from build123d import *

# Parameters (mm, degrees)
SKETCH1_R                      = 63.5
BOSS_EXTRUDE1_DEPTH            = 3.175
SKETCH2_R                      = 12.9
BOSS_EXTRUDE2_DEPTH            = 3.175
BOSS_EXTRUDE3_START            = 3.175
SKETCH3_R                      = 63.5
SKETCH3_R_2                    = 25.4
BOSS_EXTRUDE3_DEPTH            = 3.175
SKETCH5_R                      = 10.4
CUT_EXTRUDE1_DEPTH             = 2.35
SKETCH6_R                      = 5
CUT_EXTRUDE2_DEPTH             = 4
CBORE_FOR_M2_SHCS1_D           = 2.2
CBORE_FOR_M2_SHCS1_DEPTH       = 6
CBORE_FOR_M2_SHCS1_CBORE_D     = 4.4
CBORE_FOR_M2_SHCS1_CBORE_DEPTH = 2
CBORE_FOR_M2_SHCS1_TIP         = 0.660946681


with BuildPart() as part:
    # Sketch1 → Boss-Extrude1 (new body)
    with BuildSketch(Plane(origin=(0, 0, 0), x_dir=(1, 0, 0), z_dir=(0, 1, 0))):
        with Locations(Location((0, 0, 0), (0, 0, 270))):
            Circle(SKETCH1_R)
    extrude(amount=BOSS_EXTRUDE1_DEPTH)

    # Sketch2 → Boss-Extrude2 (add)
    with BuildSketch(Plane.XZ):
        with Locations(Location((0, 0, 0), (0, 0, 270))):
            Circle(SKETCH2_R)
    extrude(amount=BOSS_EXTRUDE2_DEPTH)

    # Sketch3 → Boss-Extrude3 (add)
    with BuildSketch(Plane.XZ.offset(BOSS_EXTRUDE3_START)):
        with Locations(Location((0, 0, 0), (0, 0, 270))):
            Circle(SKETCH3_R)
        with Locations(Location((0, 0, 0), (0, 0, 270))):
            Circle(SKETCH3_R_2, mode=Mode.SUBTRACT)
    extrude(amount=-BOSS_EXTRUDE3_DEPTH)

    # Sketch5 → Cut-Extrude1 (cut)
    with BuildSketch(Plane(origin=(0, 3.175, 0), x_dir=(1, 0, 0), z_dir=(0, 1, 0))):
        with Locations(Location((0, 0, 0), (0, 0, 270))):
            Circle(SKETCH5_R)
    extrude(amount=-CUT_EXTRUDE1_DEPTH, mode=Mode.SUBTRACT)

    # Sketch6 → Cut-Extrude2 (cut)
    with BuildSketch(Plane(origin=(0, 0.825, 0), x_dir=(1, 0, 0), z_dir=(0, 1, 0))):
        with Locations(Location((0, 0, 0), (0, 0, 270))):
            Circle(SKETCH6_R)
    extrude(amount=-CUT_EXTRUDE2_DEPTH, mode=Mode.SUBTRACT)

    # CBORE for M2 SHCS1
    with Locations(Plane(origin=(0, 0.825, 0), x_dir=(1, 0, 0), z_dir=(0, 1, 0))):
        with Locations((-5.65685425, 5.65685425), (0, 8), (5.65685425, 5.65685425), (8, 0), (5.65685425, -5.65685425), (0, -8), (-5.65685425, -5.65685425), (-8, 0)):
            CounterBoreHole(CBORE_FOR_M2_SHCS1_D / 2, CBORE_FOR_M2_SHCS1_CBORE_D / 2, CBORE_FOR_M2_SHCS1_CBORE_DEPTH, depth=CBORE_FOR_M2_SHCS1_DEPTH)
            with Locations((0, 0, -(CBORE_FOR_M2_SHCS1_DEPTH + CBORE_FOR_M2_SHCS1_TIP / 2))):  # 118° drill point
                Cone(0, CBORE_FOR_M2_SHCS1_D / 2, CBORE_FOR_M2_SHCS1_TIP, mode=Mode.SUBTRACT)


solid = part.part
Design review of the part built by this model. Coordinates are the model's own, in mm. A direction names the side the tool comes from. Round coordinates to 2 decimals unless told otherwise and drop trailing zeros. Write each loop counter-clockwise with the first axis right and the second up, starting at its lowest first coordinate (ties: lowest second). Pieces come first, ordered by that corner, then holes. Notation, with made-up numbers: M 2,0 L 59,0 A18 cw 59,9 Z; hole C 34.25,8 d11. An arc over 180 degrees is marked long. One line per item, written item: value. Start each with the question number.
1. Take a section at A-A on x = -17. State the section outline as (y, z) points (3 decimals), then the cut area to 3 significant figures.
2. Take a section at D-D on x = -31. State the section outline as (y, z) points (3 decimals).
3. To check wall thickness, follow probe 1 along X at (y, z) = (-1, -4.5); probe 2 along X at (y, z) = (-1.75, -9); probe 3 along X at (y, z) = (-2.7, -8). State the ranges of each line that lie inside material, in increasing order. Write a range as from..to.
4. Take a section at C-C on z = 31.5. State the section outline as (x, y) points (3 decimals), then the cut area to 3 significant figures.
5. For faces 1 (the face through (-1, -1.175, -9)), 2 (the face through (-4.88, -1.15, -1.08)), 3 (the face through (-15.456, -1.61, 20.157)), list the 3-axis set-ups (+Z, -Z, +X, -X, +Y, -Y) from which the entire face can be reached by the end or side of a thin tool; tool diameter is ignored.
6. Take a section at B-B on z = 15.5. State the section outline as (x, y) points (3 decimals).
7. Clearance check with flat-ended pins moving along their axes: P1, Ø1, axis at x = 15.5, y = 0, coming from the +Z side; P2, Ø2, axis at x = -12.5, y = 0.5, coming from the -Z side; P3, Ø6, axis at x = 0, z = -3.5, coming from the +Y side (3 decimals); P4, Ø1.8, axis at x = -5.66, z = -5.66, coming from the +Y side. State where each tip first meets the part, or that it passes through.
8. Draft analysis for pull direction X (two halves, no side actions). For faces 4 (the face through (-13, 3.175, -1)), 5 (the face through (7, -1.175, 7)), state which applies: pulls with the +X half, pulls with the -X half, needs draft (parallel to the pull), parting line crosses it, or undercut.
Computed:
1. outline: M -3.175,-61.182 L 3.175,-61.182 L 3.175,61.182 L -3.175,61.182 L -3.175,18.872 L 0,18.872 L 0,-18.872 L -3.175,-18.872 Z
1. area: 657 mm²
2. outline: M -3.175,-55.419 L 3.175,-55.419 L 3.175,55.419 L -3.175,55.419 Z
3. probe 1: x = -63.34..-25, -12.09..-7.53, -3.79..-2.18, 2.18..3.79, 7.53..12.09, 25..63.34
3. probe 2: x = -62.86..-23.75, -9.24..-0.46, 0.46..9.24, 23.75..62.86
3. probe 3: x = -62.99..-24.11, -10.12..-1.1, 1.1..10.12, 24.11..62.99
4. outline: M -55.136,-3.175 L 55.136,-3.175 L 55.136,3.175 L -55.136,3.175 Z
4. area: 700 mm²
5. face 1: +Y
5. face 2: +Y, -Y
5. face 3: -Y
6. outline: M -61.579,-3.175 L -20.122,-3.175 L -20.122,0 L 20.122,0 L 20.122,-3.175 L 61.579,-3.175 L 61.579,3.175 L -61.579,3.175 Z
7. P1: stops at z = 61.7
7. P2: stops at z = -62.45
7. P3: stops at y = 0.825
7. P4: passes through
8. face 4: needs draft
8. face 5: undercut
